Geometry check sheet. Reference: the model listing, model coordinates, mm. Face numbers are marked on the shaded views. Round coordinates to 2 decimals unless told otherwise and drop trailing zeros. Write each loop counter-clockwise with the first axis right and the second up, starting at its lowest first coordinate (ties: lowest second). Pieces come first, ordered by that corner, then holes. Notation, with made-up numbers: (10.25, 8.25) - (39.25, 8.25) arc R16 ccw to (39.25, 16.25) - close; hole circle Ø10 at (14.25, 30). An arc over 180 degrees is marked (long way). One line per question, with ' | ' between items. Start each with the question number.
from build123d import *

# Parameters (mm, degrees)
SKETCH_1_R      = 4.5
SKETCH_1_R_2    = 1.75
EXTRUDE_1_DEPTH = 3
FILLET_1_R      = 10


with BuildPart() as part:
    # Эскиз1 → Бобышка-Вытянуть1 (new body)
    # profile 1 of 2: a face of its own
    with BuildSketch(Plane.XY):
        Circle(SKETCH_1_R)
        Circle(SKETCH_1_R_2, mode=Mode.SUBTRACT)
    # profile 2 of 2: a face of its own
    with BuildSketch(Plane.XY):
        with Locations((8, 0)):
            Circle(SKETCH_1_R)
        with Locations((8, 0)):
            Circle(SKETCH_1_R_2, mode=Mode.SUBTRACT)
    extrude(amount=EXTRUDE_1_DEPTH)

    # Скругление1
    fillet_1_edges = [part.edges().sort_by_distance(p)[0] for p in [
        (4, 2.061552813, 1.5),
        (4, -2.061552813, 1.5),
    ]]
    fillet(fillet_1_edges, radius=FILLET_1_R)


solid = part.part
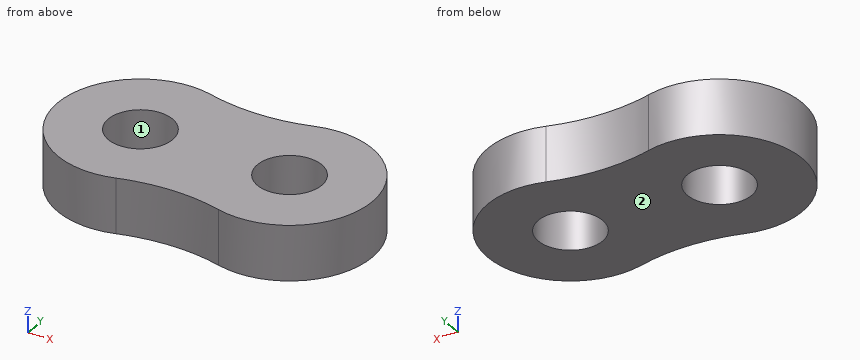
Q1. Section check A-A, the plane y = 0. Record the cut outline in (x, z).
Q2. Draft check along X on the marked faces 1 and 2. Enter one of: pulls with the +X half, pulls with the -X half, needs draft (parallel to the pull), parting line crosses it, or undercut.
Q3. Section check D-D, the plane x = 9. Record the cut outline in (y, z), then the cut area to 3 significant figures.
Q4. Section check B-B, the plane x = 0. Record the cut outline in (y, z), then the cut area to 3 significant figures.
Q5. Section check C-C, the plane y = -1.5. Record the cut outline in (x, z), then the cut area to 3 significant figures.
Q6. Go/stop test with flat-tipped pins: P1, Ø1, axis at y = 3, z = 1, coming from the -X side; P2, Ø1, axis at y = -3.5, z = 0.5, coming from the +X side. Record where each tip stops, or that it passes through.
Q7. Thickness scan on line 1 (Y direction, x = 8, z = 1.9); line 2 (X direction, y = -0.5, z = 0.35); line 3 (X direction, y = 0.75, z = 2.05). Record the ranges inside material, lowest first.
Result sheet:
1) outline: (-4.5, 0) - (-1.75, 0) - (-1.75, 3) - (-4.5, 3) - close; (1.75, 0) - (6.25, 0) - (6.25, 3) - (1.75, 3) - close; (9.75, 0) - (12.5, 0) - (12.5, 3) - (9.75, 3) - close
2) face 1: undercut | face 2: needs draft
3) outline: (-4.39, 0) - (-1.44, 0) - (-1.44, 3) - (-4.39, 3) - close; (1.44, 0) - (4.39, 0) - (4.39, 3) - (1.44, 3) - close | area: 17.7 mm²
4) outline: (-4.5, 0) - (-1.75, 0) - (-1.75, 3) - (-4.5, 3) - close; (1.75, 0) - (4.5, 0) - (4.5, 3) - (1.75, 3) - close | area: 16.5 mm²
5) outline: (-4.24, 0) - (-0.9, 0) - (-0.9, 3) - (-4.24, 3) - close; (0.9, 0) - (7.1, 0) - (7.1, 3) - (0.9, 3) - close; (8.9, 0) - (12.24, 0) - (12.24, 3) - (8.9, 3) - close | area: 38.6 mm²
6) P1: x = -3.74 | P2: x = 11.35
7) line 1: -4.5 to -1.75, 1.75 to 4.5 | line 2: -4.47 to -1.68, 1.68 to 6.32, 9.68 to 12.47 | line 3: -4.44 to -1.58, 1.58 to 6.42, 9.58 to 12.44
